Source: CAD feature listing. Evaluate the final solid. Frame: model axes, mm. A direction names the side the tool comes from. Round coordinates to 2 decimals unless told otherwise and drop trailing zeros. Write each loop counter-clockwise with the first axis right and the second up, starting at its lowest first coordinate (ties: lowest second). Pieces come first, ordered by that corner, then holes.
from build123d import *

# Parameters (mm, degrees)
F1_DEPTH = 25
F2_R     = 40
F3_SIZE  = 100
F4_R     = 120
F5_R     = 60


with BuildPart() as f1:
    # F0 (on Right) → F1 (new body)
    with BuildSketch(Plane.YZ):
        Polygon((0, 180), (0, 0), (800, 0), (800, 1684.6011072401), (406.6603498154, 2077.9407574247), (-82.4134505515, 1973.9849120159), (0, 1770.0044640112), (424.3654835952, 1594.226525303), (194.7554241761, 1039.8988057963), (-40, 990), (-40, 890), (80, 770), (80, 260), align=None)
    extrude(amount=F1_DEPTH)

    # F2
    f2_edges = [f1.edges().sort_by_distance(p)[0] for p in [
        (12.5, 194.755424, 1039.898806),
        (12.5, 0, 1770.004464),
        (12.5, -82.413451, 1973.984912),
        (12.5, 406.66035, 2077.940757),
        (12.5, 800, 1684.601107),
        (12.5, -40, 990),
        (12.5, -40, 890),
        (12.5, 80, 770),
        (12.5, 80, 260),
        (12.5, 0, 180),
    ]]
    fillet(f2_edges, radius=F2_R)

    # F3
    f3_edges = [f1.edges().sort_by_distance(p)[0] for p in [
        (12.5, 424.365484, 1594.226525),
    ]]
    chamfer(f3_edges, length=F3_SIZE)

    # F4
    f4_edges = [f1.edges().sort_by_distance(p)[0] for p in [
        (12.5, 386.09714, 1501.838572),
    ]]
    fillet(f4_edges, radius=F4_R)

    # F5
    f5_edges = [f1.edges().sort_by_distance(p)[0] for p in [
        (12.5, 331.97753, 1632.494869),
    ]]
    fillet(f5_edges, radius=F5_R)


solid = f1.part
1) Section query B-B on x = 7.75. Return the cut outline in (y, z).
Taken from the geometry:
outline: (-64.56, 1929.79) - (-6.28, 1785.56) arc R40 ccw to (15.5, 1763.59) - (309.02, 1642.01) arc R60 cw to (341.49, 1609.53) - (367.08, 1547.76) arc R120 cw to (367.08, 1455.92) - (202.81, 1059.34) arc R40 cw to (174.17, 1035.52) - (-8.32, 996.73) arc R40 ccw to (-40, 957.61) - (-40, 906.57) arc R40 ccw to (-28.28, 878.28) - (68.28, 781.72) arc R40 cw to (80, 753.43) - (80, 276.57) arc R40 cw to (68.28, 248.28) - (11.72, 191.72) arc R40 ccw to (0, 163.43) - (0, 0) - (800, 0) - (800, 1668.03) arc R40 ccw to (788.28, 1696.32) - (422.02, 2062.58) arc R40 ccw to (385.42, 2073.43) - (-35.79, 1983.9) arc R40 ccw to start
2) Pull-direction query (Z, two-part tool) for faces 3 (the face through (12.325, -35.828, 1858.681)), 4 (the face through (25, 457, 1052)), 5 (the face through (12.325, 177.764, 2029.287)); classes: released by +Z, released by -Z, zero draft, split by the parting line, or undercut.
Taken from the geometry:
face 3: undercut
face 4: zero draft
face 5: released by +Z
3) Section query D-D on y = 116. Return the cut outline in (x, z).
Taken from the geometry:
outline: (0, 0) - (25, 0) - (25, 1023.16) - (0, 1023.16) - close; (0, 1721.96) - (25, 1721.96) - (25, 2016.16) - (0, 2016.16) - close
4) Contact query for flat-ended pins moving along their axis: P1, Ø3, axis at y = 568.5, z = 768.5, coming from the -X side; P2, Ø1.5, axis at x = 2.5, y = 574.5, coming from the +Z side; P3, Ø7.5, axis at x = 17.5, z = 923.5, coming from the -Y side; P4, Ø1.5, axis at x = 7, y = 326.5, coming from the +Z side. Output: stop coordinate, or through.
Taken from the geometry:
P1: stops at x = 0
P2: stops at z = 1910.85
P3: stops at y = -40
P4: stops at z = 2061.06
5) Section query A-A on y = 258. Return the cut outline in (x, z), then the cut area to 3 significant figures.
Taken from the geometry:
outline: (0, 0) - (25, 0) - (25, 1192.58) - (0, 1192.58) - close; (0, 1663.14) - (25, 1663.14) - (25, 2046.34) - (0, 2046.34) - close
area: 39,400 mm2
6) Section query C-C on z = 850.5. Return the cut outline in (x, y), then the cut area to 3 significant figures.
Taken from the geometry:
outline: (0, -0.5) - (25, -0.5) - (25, 800) - (0, 800) - close
area: 20,000 mm2
7) Material intervals for line 1 (Z direction, x = 4, y = 81); line 2 (Y direction, x = 3.75, z = 641); line 3 (Z direction, x = 18.5, y = 331.5), sorted ascending.
Taken from the geometry:
line 1: z = 0 to 1015.72, 1736.45 to 2008.72
line 2: y = 80 to 800
line 3: z = 0 to 1370.03, 1625.75 to 2061.96
8) Reachability of faces 1 (the face through (12, 19, 831)), 2 (the face through (12.3, 607.7, 1876.9)) from +Z, -Z, +X, -X, +Y, -Y: full face, straight path, thin tool, end or side. Return the list, or none.
Taken from the geometry:
face 1: +X, -X, -Y
face 2: +Z, +X, -X, +Y
